```python
from build123d import *

# Parameters (mm, degrees)
F1_DEPTH = 19.05
F3_D     = 7.5438
F3_DEPTH = 25.4
F3_TIP   = 2.2663861689


# Not quite as in the source:
# - a pattern or mirror of a feature is missing from the dataset's text; its kind, count and spacing are read off the source's solid


with BuildPart() as f1:
    # F0 (on Right) → F1 (new body, symmetric)
    with BuildSketch(Plane.YZ):
        with BuildLine():
            Line((31.242, 19.558), (31.242, 0))
            ThreePointArc((31.242, 0), (0, -31.242), (-31.242, 0))
            Line((-31.242, 0), (-31.242, 19.558))
            Line((-31.242, 19.558), (-50.8, 19.558))
            Line((-50.8, 19.558), (-50.8, -39.1922))
            Line((-50.8, -39.1922), (0, -39.1922))
            Line((0, -39.1922), (50.8, -39.1922))
            Line((50.8, -39.1922), (50.8, 19.558))
            Line((50.8, 19.558), (31.242, 19.558))
        make_face()
    extrude(amount=F1_DEPTH, both=True)

    # F3
    with Locations(Plane(origin=(0, 50.8, 0), x_dir=(-1, 0, 0), z_dir=(0, 1, 0))):
        with Locations((0, 0)):
            f3 = Hole(F3_D / 2, depth=F3_DEPTH)
            with Locations((0, 0, -(F3_DEPTH + F3_TIP / 2))):  # 118° drill point
                Cone(0, F3_D / 2, F3_TIP, mode=Mode.SUBTRACT)

    # F3_copies: F3 across plane
    add(f3.mirror(Plane(origin=(0, 0, 0), x_dir=(0, 0, -1), z_dir=(0, -1, 0))), mode=Mode.SUBTRACT)


solid = f1.part
```
Input: part model. Units: mm. Frame: model coordinates. A direction names the side the tool comes from. Coordinates: 2 decimals unless noted, no trailing zeros. Write each loop counter-clockwise with the first axis right and the second up, starting at its lowest first coordinate (ties: lowest second). Pieces come first, ordered by that corner, then holes. Notation, with made-up numbers: (83.25, 52.25) -> (131.25, 52.25) arc R11 cw to (131.25, 56.25) -> close; hole circle Ø1 at (34.25, -24). An arc over 180 degrees is marked (long way). Answer as a JSON object with one key per item and string values.
1. Access query for faces 1 (the face through (0, 31.242, 10)), 2 (the face through (0, 41, 19.558)). Directions: +Z, -Z, +X, -X, +Y, -Y. A direction counts if a zero-diameter tool reaches every point of the face in a straight line with its end or side. Return the directions, or none.
Result set:
{"face 1": "+Z, +X, -X", "face 2": "+Z, +X, -X, +Y, -Y"}
2. Section A-A on x = 0. Return the cut outline in (y, z), then the cut area to 3 significant figures.
Result set:
{"outline": "(-50.8, -39.19) -> (50.8, -39.19) -> (50.8, -3.77) -> (31.01, -3.77) arc R31.24 cw to (-31.01, -3.77) -> (-50.8, -3.77) -> close; (-50.8, 3.77) -> (-31.24, 3.77) -> (-31.24, 19.56) -> (-50.8, 19.56) -> close; (31.24, 3.77) -> (50.8, 3.77) -> (50.8, 19.56) -> (31.24, 19.56) -> close", "area": "2,920 mm2"}
3. Section D-D on x = 7.5. Return the cut outline in (y, z).
Result set:
{"outline": "(-50.8, -39.19) -> (50.8, -39.19) -> (50.8, 19.56) -> (31.24, 19.56) -> (31.24, 0) arc R31.24 cw to (-31.24, 0) -> (-31.24, 19.56) -> (-50.8, 19.56) -> close"}
4. Section B-B on z = 14.5. Return the cut outline in (x, y).
Result set:
{"outline": "(-19.05, -50.8) -> (19.05, -50.8) -> (19.05, -31.24) -> (-19.05, -31.24) -> close; (-19.05, 31.24) -> (19.05, 31.24) -> (19.05, 50.8) -> (-19.05, 50.8) -> close"}
5. Section C-C on z = 2. Return the cut outline in (x, y).
Result set:
{"outline": "(-19.05, -50.8) -> (-3.2, -50.8) -> (-3.2, -31.24) -> (-19.05, -31.24) -> close; (-19.05, 31.24) -> (-3.2, 31.24) -> (-3.2, 50.8) -> (-19.05, 50.8) -> close; (3.2, -50.8) -> (19.05, -50.8) -> (19.05, -31.24) -> (3.2, -31.24) -> close; (3.2, 31.24) -> (19.05, 31.24) -> (19.05, 50.8) -> (3.2, 50.8) -> close"}
6. Material intervals for line 1 (Z direction, x = 0, y = -38); line 2 (Y direction, x = 16, z = 12); line 3 (X direction, y = -36.75, z = 0), sorted ascending. Write a range as from..to.
Result set:
{"line 1": "z = -39.19..-3.77, 3.77..19.56", "line 2": "y = -50.8..-31.24, 31.24..50.8", "line 3": "x = -19.05..-3.77, 3.77..19.05"}
7. Mould query, pull axis X, two halves, no side actions, for faces 3 (the face through (-19.05, -1, -36)), 4 (the face through (-2.99, 40.77, -2.3)), 5 (the face through (0, -41, 19.558)). Classes: released by +X, released by -X, zero draft, split by the parting line, or undercut.
Result set:
{"face 3": "released by -X", "face 4": "undercut", "face 5": "zero draft"}
